Could you check a few things on this model? Use its own coordinates, in mm. A direction names the side the tool comes from. Give positions to 0.01 mm unless a question says otherwise; leave off trailing zeros. Order: outer loops, then holes, each group sorted by start corner. A loop starts at its lowest first (then second) coordinate and runs counter-clockwise, first axis right, second up. Notation, with made-up numbers: (-19, 53) -> (-12, 53) arc R31 ccw to (-12, 90) -> close; hole circle Ø1 at (39, 9). An arc over 180 degrees is marked (long way). Write each question's results on one line, items separated by ' | '.
```python
from build123d import *

# Parameters (mm, degrees)
SKETCH2_W           = 85
SKETCH2_H           = 85
SKETCH3_W           = 65
SKETCH3_H           = 65
SKETCH10_W          = 17
SKETCH10_H          = 17
BOSS_EXTRUDE5_DEPTH = 57.5
SKETCH11_W          = 15
SKETCH11_H          = 3.5
CUT_EXTRUDE1_DEPTH  = 25
BOSS_EXTRUDE6_START = -5.75
BOSS_EXTRUDE6_DEPTH = 6


with BuildPart() as part:
    # Sketch2 → Loft1 section 0
    with BuildSketch(Plane(origin=(0, 0, 0), x_dir=(1, 0, 0), z_dir=(0, 1, 0))):
        Rectangle(SKETCH2_W, SKETCH2_H)
    # Sketch3 → Loft1 section 1
    with BuildSketch(Plane(origin=(0, 7.5, 0), x_dir=(1, 0, 0), z_dir=(0, 1, 0))):
        with Locations((-10, 0)):
            Rectangle(SKETCH3_W, SKETCH3_H)
    loft()

    # Sketch10 → Boss-Extrude5 (add)
    with BuildSketch(Plane(origin=(0, 7.5, 0), x_dir=(1, 0, 0), z_dir=(0, 1, 0))):
        with Locations((-34, 0)):
            Rectangle(SKETCH10_W, SKETCH10_H)
    extrude(amount=BOSS_EXTRUDE5_DEPTH)

    # Sketch11 → Cut-Extrude1 (cut)
    with BuildSketch(Plane(origin=(0, 65, 0), x_dir=(1, 0, 0), z_dir=(0, 1, 0))):
        with Locations((-34, 5.75)):
            Rectangle(SKETCH11_W, SKETCH11_H)
        with Locations((-34, -5.75)):
            Rectangle(SKETCH11_W, SKETCH11_H)
    extrude(amount=-CUT_EXTRUDE1_DEPTH, mode=Mode.SUBTRACT)

    # Sketch14 → Boss-Extrude6 (add)
    with BuildSketch(Plane.XY.offset(8.5).offset(BOSS_EXTRUDE6_START)):
        Polygon((-25.5, 32.5), (-11.06624327, 7.5), (-25.5, 7.5), align=None)
    extrude(amount=-BOSS_EXTRUDE6_DEPTH)


solid = part.part
```
Q1. For faces 5 (the flat face through (-34, 36, 8.5)), 6 (the flat face through (-34, 65, -2)), 7 (the flat face through (-21, 15, 2.75)), 8 (the flat face through (-41.5, 53, -6)), which set-ups out of +Z, -Z, +X, -X, +Y, -Y let a thin tool reach every point of the face, with its end or its side?
Here are the results:
face 5: +Z, +X, -X, +Y | face 6: +Z, -Z, +X, -X, +Y | face 7: +Z, +X, +Y | face 8: +Y
Q2. Suppose I cut it at A-A on y = 49.5. Please give me the cut outline in (x, z), and give its area (3 significant figures).
Here are the results:
outline: (-42.5, -8.5) -> (-25.5, -8.5) -> (-25.5, 8.5) -> (-42.5, 8.5) -> close; hole (-41.5, -7.5) -> (-26.5, -7.5) -> (-26.5, -4) -> (-41.5, -4) -> close; hole (-41.5, 4) -> (-26.5, 4) -> (-26.5, 7.5) -> (-41.5, 7.5) -> close | area: 184 mm²
Q3. I need wall thicknesses on line 1 along Y through (x, z) = (17, -13.5); line 2 along Z through (x, y) = (-36.5, 32.5); line 3 along X through (y, z) = (56.5, 1). Which ranges of each line are inside material? Lowest first, please.
Here are the results:
line 1: y = 0 to 7.5 | line 2: z = -8.5 to 8.5 | line 3: x = -42.5 to -25.5
Q4. Thinking about a two-plate mould opening in X: for faces 1 (the flat face through (-34, 40, -6)), 2 (the flat face through (-34, 36, -8.5)), 3 (the flat face through (-25.5, 36, 0)), 4 (the flat face through (-42.5, 23, 0)), which applies, +X half, -X half, draft (parallel to the pull), parting line (faces both ways), or undercut?
Here are the results:
face 1: undercut | face 2: draft | face 3: +X half | face 4: -X half
Q5. Suppose I cut it at C-C on y = 26. Please give me the cut outline in (x, z).
Here are the results:
outline: (-42.5, -8.5) -> (-25.5, -8.5) -> (-25.5, -3.25) -> (-21.75, -3.25) -> (-21.75, 2.75) -> (-25.5, 2.75) -> (-25.5, 8.5) -> (-42.5, 8.5) -> close
Q6. I'm going to push flat-ended pins straight in: pin 1 Ø8 at (x, z) = (12, -4) entering from +Y; pin 2 Ø4 at (x, z) = (-9, -26) entering from -Y; pin 3 Ø12 at (x, y) = (-31.5, 58.5) entering from -Z; pin 4 Ø8.5 at (y, z) = (42, 1.5) entering from +X. Where does each tip first touch, or does it pass through?
Here are the results:
pin 1: stops at y = 7.5 | pin 2: stops at y = 0 | pin 3: stops at z = -8.5 | pin 4: stops at x = -25.5
Q7. Suppose I cut it at B-B on y = 11. Please give me the cut outline in (x, z), and give its area (3 significant figures).
Here are the results:
outline: (-42.5, -8.5) -> (-25.5, -8.5) -> (-25.5, -3.25) -> (-13.09, -3.25) -> (-13.09, 2.75) -> (-25.5, 2.75) -> (-25.5, 8.5) -> (-42.5, 8.5) -> close | area: 363 mm²
